Input: part model. Units: mm. Frame: model coordinates. Face numbers are marked on the shaded views. Give positions to 0.01 mm unless a question says otherwise; leave off trailing zeros. Loops run counter-clockwise (first coordinate to the right, second up) from the corner with the lowest first, then second, coordinate; pieces in that order, holes last. Notation, with made-up numbers: (45, 69.5) - (100, 69.5) arc R10 ccw to (100, 85.5) - close; hole circle Ø2 at (31, 17.5). An arc over 180 degrees is marked (long way). Answer as a JSON object with one key per item and string values.
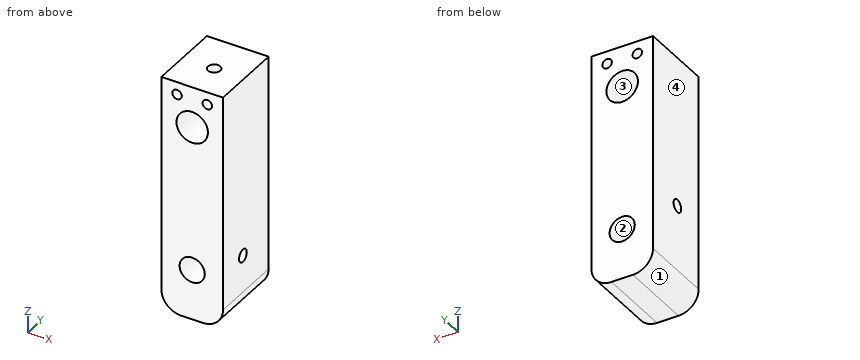
Autodesk Inventor part; units mm, degrees
ref_plane "YZ Plane" through (0, 0, 0) normal (1, 0, 0) x (0, 1, 0)
ref_plane "XZ Plane" through (0, 0, 0) normal (0, 1, 0) x (-1, 0, 0)
ref_plane "XY Plane" through (0, 0, 0) normal (0, 0, 1) x (1, 0, 0)
sketch "Sketch1" plane through (0, 0, 0) normal (0, 1, 0) x (-1, 0, 0)
  line L0 (-5.3975, -59.69) -> (5.3975, -59.69)
  line L1 (15.5575, -49.53) -> (15.5575, 59.69)
  line L2 (15.5575, 59.69) -> (-15.5575, 59.69)
  line L3 (-15.5575, 59.69) -> (-15.5575, -49.53)
  line L4 (-15.5575, -59.69) -> (15.5575, 59.69) construction
  line L5 (15.5575, -59.69) -> (-15.5575, 59.69) construction
  arc A0 (5.3975, -59.69) -> (15.5575, -49.53) centre (5.3975, -49.53) ccw
  arc A1 (-15.5575, -49.53) -> (-5.3975, -59.69) centre (-5.3975, -49.53) ccw
  circle A2 centre (0, 39.0525) radius 7.9375
  line L6 (0, -93.6381) -> (0, 115.0739)
  circle A3 centre (7.62, 53.34) radius 2.3813
  circle A4 centre (-7.62, 53.34) radius 2.3813
  point P0 (0, 0)
  point P1 (0, 0)
  dimension "d0" = 119.38
  dimension "d1" = 31.115
  dimension "d2" = 10.16
  dimension "d3" = 15.875
  dimension "d4" = 20.6375
  dimension "d51" = 4.7625
  dimension "d52" = 15.24
  dimension "d53" = 6.35
extrude "Extrusion1" add sketch "Sketch1" along normal blind 37.719 contours A1 L3 L2 L6 A2 L0 | L6 A2 L2 L1 A0 L0
sketch "Sketch2" plane through (0, 37.719, 0) normal (0, 1, 0) x (1, 0, 0)
  line L0 (5.3975, 59.69) -> (-5.3975, 59.69)
  point P0 (0, 0)
  point P1 (0, 34.29)
  dimension "d7" = 25.4
hole "Hole1" at (0, 37.719, -34.29) direction (0, -1, 0) diameter 12.7 end through all
hole "Hole3" at (0.3897, 17.4911, 59.69) direction (0, 0, -1) diameter 6.35 depth 12.7 tip angle 118
hole "Hole4" at (-15.5575, 17.5708, -16.4401) direction (1, 0, 0) diameter 6.35 depth 12.7 tip angle 118
hole "Hole5" at (15.5575, 16.4302, -30.8144) direction (-1, 0, 0) diameter 6.35 depth 12.7 tip angle 118
properties part number "Fixture_Base"
Item 1: Contact query for a flat-ended pin moving along its axis: P1, Ø8, axis at x = 11.5, y = 26.5, coming from the -Z side. Output: stop coordinate, or through.
Geometry check:
{"P1": "stops at z = -59.47"}
Item 2: Cut plane A-A (x = -12.5). Return loops of the section in (y, z) (3 decimals), then the cut area to 3 significant figures.
Geometry check:
{"outline": "(0, -56.795) - (37.719, -56.795) - (37.719, 59.69) - (0, 59.69) - close; hole circle Ø6.35 at (17.571, -16.44)", "area": "4,360 mm2"}
Item 3: Mould query, pull axis Z, two halves, no side actions, for the marked faces 1, 2, 3 and 4. Classes: released by +Z, released by -Z, zero draft, split by the parting line, or undercut.
Geometry check:
{"face 1": "released by -Z", "face 2": "undercut", "face 3": "undercut", "face 4": "zero draft"}
Item 4: Material intervals for line 1 (X direction, y = 24, z = 53); line 2 (Z direction, x = 0, y = 22.5) (3 decimals); line 3 (Y direction, x = -3, z = -16.5), sorted ascending. Write a range as [from, to].
Geometry check:
{"line 1": "x = [-15.56, -9.98], [-5.26, 5.26], [9.98, 15.56]", "line 2": "z = [-59.69, -40.64], [-27.94, 31.115], [46.99, 59.69]", "line 3": "y = [0, 14.4], [20.75, 37.72]"}
Item 5: Cut plane B-B (y = 34.5). Give the number of separate pieces and of enclosed holes in the cut face, then the cut area to 3 significant figures.
Geometry check:
{"separate pieces": "1", "enclosed holes": "4", "area": "3,310 mm2"}
